Here's how the part is built. I have some questions about the finished solid (model axes, mm). A direction names the side the tool comes from. Round coordinates to 2 decimals unless told otherwise and drop trailing zeros. Write each loop counter-clockwise with the first axis right and the second up, starting at its lowest first coordinate (ties: lowest second). Pieces come first, ordered by that corner, then holes. Notation, with made-up numbers: (49, 48) - (103, 48) arc R10 cw to (103, 59) - close; hole circle Ø6 at (-40, 14.5). An arc over 180 degrees is marked (long way). Use one line per item in the form item = value. Start each with the question number.
1. I want a section at C-C, the plane y = 70.5. List the corners of the cut face in (x, z) for me.
2. If I drill on line 1 along Y through (x, z) = (0.9, -21); line 2 along Y through (x, z) = (2.8, 8); line 3 along Z through (x, y) = (2.3, 56), over which ranges is the centre line in solid material (lowest first)?
3. Will these pins go through, and if not, where does the flat tip stop? pin 1 (0.9 mm diameter, centred on x = 2, z = -22.5, fed in from -Y); pin 2 (0.9 mm diameter, centred on x = 2, y = 94, fed in from -Z); pin 3 (1.5 mm diameter, centred on x = 1.5, z = -22, fed in from +Y).
4. Which directions (+Z, -Z, +X, -X, +Y, -Y) give clear straight access to the entire face, cutting with the end or side of a thin tool? Please do faces 1 (the flat face through (1, 15.693, -22)), 2 (the flat face through (1, 94, -2.526)), 3 (the flat face through (1, 45.693, -22)), 4 (the flat face through (1, 91, -20.526)).
5. We'd pull the mould along Z, two halves only. Please class faces 5 (the flat face through (1, 9, -3.676)), 6 (the flat face through (1, 75.693, -22)), 7 (the flat face through (1, 81, -23.676)): +Z half, -Z half, draft (parallel to the pull), parting line (faces both ways), or undercut.
6. I want a section at B-B, the plane z = 3. List the corners of the cut face in (x, y) for me, plus the area to 3 significant figures.
```python
from build123d import *

# Parameters (mm, degrees)
SKETCH1_R           = 1.5
BOSS_EXTRUDE1_DEPTH = 3


with BuildPart() as part:
    # Sketch1 → Boss-Extrude1 (new body)
    with BuildSketch(Plane(origin=(0, 0, 0), x_dir=(0, 0, -1), z_dir=(1, 0, 0))):
        with BuildLine():
            Line((-9.38169605, 95.692985903), (-1.06418499, 95.692985903))
            Line((-1.06418499, 95.692985903), (2.525652309, 95.692985903))
            Line((2.525652309, 95.692985903), (2.525652309, 92.692985903))
            Line((2.525652309, 92.692985903), (12.525652309, 92.692985903))
            Line((12.525652309, 92.692985903), (12.525652309, 95.692985903))
            Line((12.525652309, 95.692985903), (20.525652309, 95.692985903))
            Line((20.525652309, 95.692985903), (20.525652309, 85.692985903))
            Line((20.525652309, 85.692985903), (23.675577753, 85.692985903))
            Line((23.675577753, 85.692985903), (23.675577753, 75.692985903))
            Line((23.675577753, 75.692985903), (20.675577753, 75.692985903))
            Line((20.675577753, 75.692985903), (20.675577753, 65.692985903))
            Line((20.675577753, 65.692985903), (23.675577753, 65.692985903))
            Line((23.675577753, 65.692985903), (23.675577753, 55.692985903))
            Line((23.675577753, 55.692985903), (20.675577753, 55.692985903))
            Line((20.675577753, 55.692985903), (20.675577753, 45.692985903))
            Line((20.675577753, 45.692985903), (23.675577753, 45.692985903))
            Line((23.675577753, 45.692985903), (23.675577753, 35.692985903))
            Line((23.675577753, 35.692985903), (20.675577753, 35.692985903))
            Line((20.675577753, 35.692985903), (20.675577753, 25.692985903))
            Line((20.675577753, 25.692985903), (23.675577753, 25.692985903))
            Line((23.675577753, 25.692985903), (23.675577753, 15.692985903))
            Line((23.675577753, 15.692985903), (20.675577753, 15.692985903))
            Line((20.675577753, 15.692985903), (20.675577753, 5.692985903))
            Line((20.675577753, 5.692985903), (13.675577753, 5.692985903))
            Line((13.675577753, 5.692985903), (13.675577753, 11.692985903))
            Line((13.675577753, 11.692985903), (3.675577753, 11.692985903))
            Line((3.675577753, 11.692985903), (3.675577753, 5.692985903))
            Line((3.675577753, 5.692985903), (-1.324422247, 5.692985903))
            Line((-1.324422247, 5.692985903), (-1.324422247, 82.492985903))
            Line((-1.324422247, 82.492985903), (-8.482000981, 82.492985903))
            ThreePointArc((-8.482000981, 82.492985903), (-14.479905975, 88.714837423), (-9.38169605, 95.692985903))
        make_face()
        with Locations((-7.783554384, 89.092985903)):
            Circle(SKETCH1_R, mode=Mode.SUBTRACT)
    extrude(amount=BOSS_EXTRUDE1_DEPTH)


solid = part.part
```
Model answer:
q1.outline = (0, -20.68) - (3, -20.68) - (3, 1.32) - (0, 1.32) - close
q2.line_1 = 15.69 to 25.69, 35.69 to 45.69, 55.69 to 65.69, 75.69 to 85.69
q2.line_2 = 82.49 to 87.61, 90.58 to 95.69
q2.line_3 = -23.68 to 1.32
q3.pin_1 = 15.69
q3.pin_2 = -20.53
q3.pin_3 = 85.69
q4.face_1 = -Z, +X, -X, -Y
q4.face_2 = +X, -X, +Y
q4.face_3 = -Z, +X, -X
q4.face_4 = -Z, +X, -X, +Y
q5.face_5 = undercut
q5.face_6 = draft
q5.face_7 = -Z half
q6.outline = (0, 82.49) - (3, 82.49) - (3, 95.69) - (0, 95.69) - close
q6.area = 39.6 mm2
